from build123d import *

# Parameters (mm, degrees)
SKETCH12_W          = 62.8142
SKETCH12_H          = 87.376
BOSS_EXTRUDE5_DEPTH = 3.81
SKETCH22_W          = 3.81
SKETCH22_H          = 2.54
BOSS_EXTRUDE6_DEPTH = 5.08
SKETCH23_R          = 1.1303
CUT_EXTRUDE5_DEPTH  = 5.08
SKETCH25_W          = 45.3644
SKETCH25_H          = 36.2458
CUT_EXTRUDE6_DEPTH  = 1.9304
SKETCH26_R          = 1.5
CUT_EXTRUDE7_DEPTH  = 1.9304


with BuildPart() as part:
    # Sketch12 → Boss-Extrude5 (new body)
    with BuildSketch(Plane.XY):
        Rectangle(SKETCH12_W, SKETCH12_H)
    extrude(amount=-BOSS_EXTRUDE5_DEPTH)

    # Sketch22 → Boss-Extrude6 (add)
    with BuildSketch(Plane(origin=(0, 0, -3.81), x_dir=(-1, 0, 0), z_dir=(0, 0, -1))):
        with Locations((-28.1803602, -1.397)):
            Rectangle(SKETCH22_W, SKETCH22_H)
        with Locations((28.1803602, -1.397)):
            Rectangle(SKETCH22_W, SKETCH22_H)
    extrude(amount=BOSS_EXTRUDE6_DEPTH)

    # Sketch23 → Cut-Extrude5 (cut)
    with BuildSketch(Plane(origin=(0, -0.127, 0), x_dir=(1, 0, 0), z_dir=(0, 1, 0))):
        with Locations((28.1803602, 6.35)):
            Circle(SKETCH23_R)
        with Locations((-28.362608627, 6.35)):
            Circle(SKETCH23_R)
    extrude(amount=-CUT_EXTRUDE5_DEPTH, mode=Mode.SUBTRACT)

    # Sketch25 → Cut-Extrude6 (cut)
    with BuildSketch(Plane.XY):
        with Locations((0, 20.4851)):
            Rectangle(SKETCH25_W, SKETCH25_H)
        with Locations((0, -20.4851)):
            Rectangle(SKETCH25_W, SKETCH25_H)
    extrude(amount=-CUT_EXTRUDE6_DEPTH, mode=Mode.SUBTRACT)

    # Sketch26 → Cut-Extrude7 (cut)
    with BuildSketch(Plane.XY.offset(-1.9304)):
        with Locations((19.6822, 20.608)):
            Circle(SKETCH26_R)
        with Locations((19.6822, -20.3622)):
            Circle(SKETCH26_R)
        with Locations((-19.6822, -20.3622)):
            Circle(SKETCH26_R)
        with Locations((-19.6822, 20.608)):
            Circle(SKETCH26_R)
    extrude(amount=-CUT_EXTRUDE7_DEPTH, mode=Mode.SUBTRACT)


solid = part.part
Geometry check sheet. Reference: the model listing, model coordinates, mm. A direction names the side the tool comes from. Give positions to 0.01 mm unless a question says otherwise; leave off trailing zeros. Order: outer loops, then holes, each group sorted by start corner. A loop starts at its lowest first (then second) coordinate and runs counter-clockwise, first axis right, second up. Notation, with made-up numbers: (40, -18) - (91, -18) arc R6 ccw to (91, -7) - close; hole circle Ø4 at (67, -18.5). An arc over 180 degrees is marked (long way). Answer as a JSON object with one key per item and string values.
(1) Cross-section at A-A (z = -6.35). Record the cut outline in (x, y), then the cut area to 3 significant figures.
Report:
{"outline": "(-30.09, -2.67) - (-29.49, -2.67) - (-29.49, -0.13) - (-30.09, -0.13) - close; (-27.23, -2.67) - (-26.28, -2.67) - (-26.28, -0.13) - (-27.23, -0.13) - close; (26.28, -2.67) - (27.05, -2.67) - (27.05, -0.13) - (26.28, -0.13) - close; (29.31, -2.67) - (30.09, -2.67) - (30.09, -0.13) - (29.31, -0.13) - close", "area": "7.87 mm^2"}
(2) Tool access check on faces 4 (the flat face through (-27, -2.667, -6)), 5 (the flat face through (30.085, -1, -6)), 6 (the flat face through (-22.682, 20, -1)), 7 (the flat face through (26.275, -1, -6)), 8 (the flat face through (28, -0.127, -5)). Record the directions out of +Z, -Z, +X, -X, +Y, -Y that give a thin tool (end or side, any length) a straight path to the whole face; none if there is none.
Report:
{"face 4": "-Z, +X, -X, -Y", "face 5": "-Z, +X, +Y, -Y", "face 6": "+Z", "face 7": "-Z, +Y, -Y", "face 8": "-Z, +X, -X, +Y"}
(3) Draft check along Y on faces 1 (the flat face through (-30.085, -1, -6)), 2 (the flat face through (28, -2.667, -5)), 3 (the flat face through (0, -2.362, -1)). Enter one of: released by +Y, released by -Y, zero draft, split by the parting line, or undercut.
Report:
{"face 1": "zero draft", "face 2": "released by -Y", "face 3": "undercut"}
(4) Material ranges on line 1 (Y direction, x = 4.5, z = -0.75); line 2 (X direction, y = -1.5, z = -6.35); line 3 (X direction, y = -22, z = -0.75), recorded low to high.
Report:
{"line 1": "-43.69 to -38.61, -2.36 to 2.36, 38.61 to 43.69", "line 2": "-30.09 to -29.49, -27.23 to -26.28, 26.28 to 27.05, 29.31 to 30.09", "line 3": "-31.41 to -22.68, 22.68 to 31.41"}
(5) Cross-section at B-B (z = -1). Record the cut outline in (x, y).
Report:
{"outline": "(-31.41, -43.69) - (31.41, -43.69) - (31.41, 43.69) - (-31.41, 43.69) - close; hole (-22.68, -38.61) - (22.68, -38.61) - (22.68, -2.36) - (-22.68, -2.36) - close; hole (-22.68, 2.36) - (22.68, 2.36) - (22.68, 38.61) - (-22.68, 38.61) - close"}
(6) Depth check by flat-ended pin: pin 1 Ø6 at (x, y) = (-10.5, -11) entering from +Z; pin 2 Ø1 at (x, z) = (-16, -5.5) entering from +Y; pin 3 Ø5 at (x, y) = (-11, 11.5) entering from -Z; pin 4 Ø10 at (x, y) = (-20, -24.5) entering from +Z. Enter the tip coordinate at first touch or a pass-through.
Report:
{"pin 1": "z = -1.93", "pin 2": "through", "pin 3": "z = -3.81", "pin 4": "z = 0"}
(7) Cross-section at C-C (y = -9). Record the cut outline in (x, z).
Report:
{"outline": "(-31.41, -3.81) - (31.41, -3.81) - (31.41, 0) - (22.68, 0) - (22.68, -1.93) - (-22.68, -1.93) - (-22.68, 0) - (-31.41, 0) - close"}
(8) Cross-section at D-D (x = 13). Record the cut outline in (y, z).
Report:
{"outline": "(-43.69, -3.81) - (43.69, -3.81) - (43.69, 0) - (38.61, 0) - (38.61, -1.93) - (2.36, -1.93) - (2.36, 0) - (-2.36, 0) - (-2.36, -1.93) - (-38.61, -1.93) - (-38.61, 0) - (-43.69, 0) - close"}
